Autodesk Fusion 360 part; units mm, degrees
sketch "Sketch1" plane through (0, 0, 0) normal (0, 0, 1) x (1, 0, 0)
  line L0 (0, 0) -> (30, 0)
  line L1 (30, 0) -> (30, 42)
  line L2 (30, 42) -> (0, 42)
  line L3 (0, 42) -> (0, 0)
  circle A0 centre (2, 40) radius 2
  circle A1 centre (28, 40) radius 2
  circle A2 centre (2, 14) radius 2
  circle A3 centre (28, 14) radius 2
  circle A4 centre (2, 40) radius 3
  circle A5 centre (28, 40) radius 3
  circle A6 centre (28, 14) radius 3
  circle A7 centre (2, 14) radius 3
  circle A8 centre (15, 27) radius 1.5
  dimension "d1" = 30
  dimension "d2" = 42
  dimension "d3" = 4
  dimension "d6" = 26
  dimension "d7" = -26
  dimension "d8" = 6
  dimension "d9" = 6
  dimension "d10" = 6
  dimension "d11" = 6
  dimension "d14" = 3
  dimension "d15" = 15
  dimension "d16" = 15
extrude "Extrude1" add sketch "Sketch1" along normal blind 1.75 contours L0 L1 L2 L3 A4 A5 A6 A7 | L3 A7 | L3 A7 | L1 A6 | L1 A6 | L2 L3 A4 | L2 L3 A0 A4 | L1 L2 A1 A5 | L1 L2 A5 | L2 L3 A0 | L1 L2 A1
For this review, take the finished solid that the model builds, in its own axes (mm). A direction names the side the tool comes from. Round coordinates to 2 decimals unless told otherwise and drop trailing zeros. Loops run counter-clockwise (first coordinate to the right, second up) from the corner with the lowest first, then second, coordinate; pieces in that order, holes last. Notation, with made-up numbers: (19, 79.5) - (65, 79.5) arc R21 cw to (65, 104.5) - close; hole circle Ø9 at (25.25, 30). An arc over 180 degrees is marked (long way). Use one line per item in the form item = value.
1) We need section A-A on x = 15. Write out the cut boundary in (y, z), then the cut area to 4 significant figures.
Solutions:
outline = (0, 0) - (25.5, 0) - (25.5, 1.75) - (0, 1.75) - close; (28.5, 0) - (42, 0) - (42, 1.75) - (28.5, 1.75) - close
area = 68.25 mm2
2) We need section C-C on x = 2. Write out the cut boundary in (y, z).
Solutions:
outline = (0, 0) - (12, 0) - (12, 1.75) - (0, 1.75) - close; (16, 0) - (38, 0) - (38, 1.75) - (16, 1.75) - close; (42, 0) - (43, 0) - (43, 1.75) - (42, 1.75) - close
3) Tool access review of faces 4 (the face through (0, 27, 1)), 5 (the face through (15, 22, 0)), 6 (the face through (30, 27, 1)), 7 (the face through (15, 42, 1)), 8 (the face through (30, 6, 1)): name each direction out of +Z, -Z, +X, -X, +Y, -Y from which nothing blocks a thin tool from reaching the whole face with its end or side.
Solutions:
face_4 = +Z, -Z, -X
face_5 = -Z, +X, -X, +Y, -Y
face_6 = +Z, -Z, +X
face_7 = +Z, -Z, +Y
face_8 = +Z, -Z, +X, -Y
4) Wall thickness on probe 1 along Y at (x, z) = (28, 1.1); probe 2 along X at (y, z) = (40, 1.3); probe 3 along Y at (x, z) = (1, 0.65): over which ranges is each line inside the solid? List them lowest first.
Solutions:
probe_1 = 0 to 12, 16 to 38, 42 to 43
probe_2 = -1 to 0, 4 to 26, 30 to 31
probe_3 = 0 to 12.27, 15.73 to 38.27, 41.73 to 42.83
5) We need section B-B on y = 27. Write out the cut boundary in (x, z).
Solutions:
outline = (0, 0) - (13.5, 0) - (13.5, 1.75) - (0, 1.75) - close; (16.5, 0) - (30, 0) - (30, 1.75) - (16.5, 1.75) - close
6) Clearance check with flat-ended pins moving along their axes: P1, Ø0.5, axis at y = 7, z = 1, coming from the -X side; P2, Ø3, axis at x = 2, y = 14, coming from the +Z side; P3, Ø0.5, axis at y = 23, z = 1, coming from the +X side. State where each tip first meets the part, or that it passes through.
Solutions:
P1 = 0
P2 = through
P3 = 30
7) Mouldability with a two-part tool opening along X and no side actions: class faces 1 (the face through (0, 6, 1)), 2 (the face through (15, 22, 1.75)), 3 (the face through (13.89, 25.99, 0.86)) as pulls with the +X half, pulls with the -X half, needs draft (parallel to the pull), parting line crosses it, or undercut.
Solutions:
face_1 = pulls with the -X half
face_2 = needs draft
face_3 = undercut
8) We need section D-D on z = 1.3. Write out the cut boundary in (x, y), then the cut area to 3 significant figures.
Solutions:
outline = (0, 0) - (30, 0) - (30, 11.76) arc R3 ccw to (30, 16.24) - (30, 37.76) arc R3 ccw (long way) to (25.76, 42) - (4.24, 42) arc R3 ccw (long way) to (0, 37.76) - (0, 16.24) arc R3 ccw to (0, 11.76) - close; hole circle Ø4 at (2, 14); hole circle Ø4 at (2, 40); hole circle Ø3 at (15, 27); hole circle Ø4 at (28, 14); hole circle Ø4 at (28, 40)
area = 1,220 mm2
